Source: CAD feature listing. Evaluate the final solid. Frame: model axes, mm. Give positions to 0.01 mm unless a question says otherwise; leave off trailing zeros. Write each loop counter-clockwise with the first axis right and the second up, starting at its lowest first coordinate (ties: lowest second). Pieces come first, ordered by that corner, then holes.
```python
from build123d import *

# Parameters (mm, degrees)
BOSS_EXTRUDE1_DEPTH       = 2.9972
F_8_CLEARANCE_HOLE1_D     = 4.3053
F_8_CLEARANCE_HOLE1_DEPTH = 6.351016


with BuildPart() as part:
    # Sketch1 → Boss-Extrude1 (new body)
    with BuildSketch(Plane.XY):
        with BuildLine():
            Line((-46.355, 6.35), (46.355, 6.35))
            ThreePointArc((46.355, 6.35), (52.705, 0), (46.355, -6.35))
            Line((46.355, -6.35), (-46.355, -6.35))
            ThreePointArc((-46.355, -6.35), (-52.705, 0), (-46.355, 6.35))
        make_face()
    extrude(amount=BOSS_EXTRUDE1_DEPTH)

    # #8 Clearance Hole1
    with Locations(Plane.XY.offset(2.9972)):
        with Locations((-46.355, 0), (46.355, 0)):
            Hole(F_8_CLEARANCE_HOLE1_D / 2, depth=F_8_CLEARANCE_HOLE1_DEPTH)


solid = part.part
```
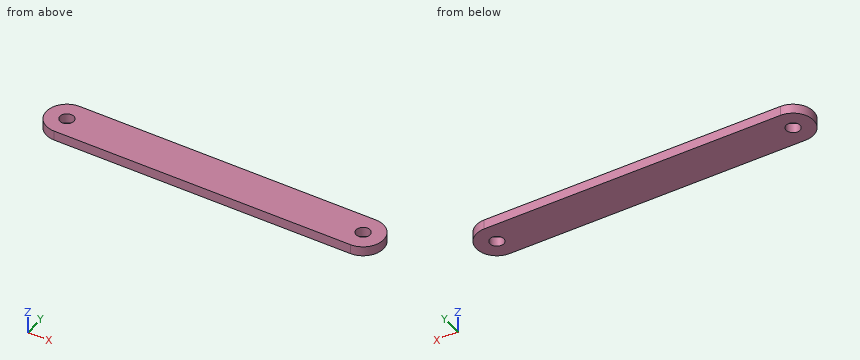
1. Section query A-A (y = 0). Return loops of the section in (x, z) (3 decimals), plus the area to 3 significant figures.
2. Section query B-B (z = 2.35). Return loops of the section in (x, y) (3 decimals).
3. Section query C-C (y = 4.5). Return loops of the section in (x, z), plus the area to 3 significant figures.
4. Pin query (flat end, axial travel): P1, Ø3.5, axis at x = 46.355, y = 0, coming from the +Z side. Return the tip coordinate at first contact, or that it passes through.
5. Line query: probe 1 along Y at (x, z) = (-46.5, 1.65); probe 2 along X at (y, z) = (-0.5, 1.75); probe 3 along X at (y, z) = (-1.5, 1.55). Output: solid intervals per line, ascending.
The answers:
1. outline: (-52.705, 0) - (-48.508, 0) - (-48.508, 2.997) - (-52.705, 2.997) - close; (-44.202, 0) - (44.202, 0) - (44.202, 2.997) - (-44.202, 2.997) - close; (48.508, 0) - (52.705, 0) - (52.705, 2.997) - (48.508, 2.997) - close
1. area: 290 mm2
2. outline: (-46.355, -6.35) - (46.355, -6.35) arc R6.35 ccw to (46.355, 6.35) - (-46.355, 6.35) arc R6.35 ccw to start; hole circle Ø4.305 at (-46.355, 0); hole circle Ø4.305 at (46.355, 0)
3. outline: (-50.84, 0) - (50.84, 0) - (50.84, 3) - (-50.84, 3) - close
3. area: 305 mm2
4. P1: passes through
5. probe 1: y = -6.35 to -2.15, 2.15 to 6.35
5. probe 2: x = -52.69 to -48.45, -44.26 to 44.26, 48.45 to 52.69
5. probe 3: x = -52.53 to -47.9, -44.81 to 44.81, 47.9 to 52.53
